```python
from build123d import *

# Parameters (mm, degrees)
CUT_EXTRUDE1_DEPTH  = 2
CUT_EXTRUDE1_DRAFT  = -12
SKETCH3_R           = 1.5
BOSS_EXTRUDE1_DEPTH = 36


with BuildPart() as part:
    # Sketch1 → Revolve2 (revolve)
    with BuildSketch(Plane(origin=(0, 0, 0), x_dir=(1, 0, 0), z_dir=(0, 1, 0))):
        with BuildLine():
            Line((0, 0), (0, 2))
            Line((0, 2), (1.798285661, 2))
            ThreePointArc((1.798285661, 2), (1.941964308, 1.978911731), (2.07352322, 1.917425786))
            ThreePointArc((2.07352322, 1.917425786), (2.674697589, 1.044998208), (2.5, 0))
            Line((2.5, 0), (0, 0))
        make_face()
    revolve(axis=Axis((0, 0, -0.65925001), (0, 0, -1)))


with BuildPart() as cut_extrude1_tool:
    # Sketch2 → Cut-Extrude1 (with draft: the straight prism first)
    with BuildSketch(Plane(origin=(0, 0, -2), x_dir=(-1, 0, 0), z_dir=(0, 0, -1))):
        Polygon((0.5, -0.5), (2, -0.5), (2, 0.5), (0.5, 0.5), (0.5, 2), (-0.5, 2), (-0.5, 0.5), (-2, 0.5), (-2, -0.5), (-0.5, -0.5), (-0.5, -2), (0.5, -2), align=None)
    extrude(amount=-CUT_EXTRUDE1_DEPTH)
    # Cut-Extrude1: the draft: its side faces are tilted about the plane it starts from
    cut_extrude1_sides = [cut_extrude1_tool.faces().sort_by_distance(p)[0] for p in [
        (-1.25, -0.5, -1),
        (-2, 0, -1),
        (-1.25, 0.5, -1),
        (-0.5, 1.25, -1),
        (0, 2, -1),
        (0.5, 1.25, -1),
        (1.25, 0.5, -1),
        (2, 0, -1),
        (1.25, -0.5, -1),
        (0.5, -1.25, -1),
        (0, -2, -1),
        (-0.5, -1.25, -1),
    ]]
    draft(cut_extrude1_sides, Plane(origin=(0, 0, -2), x_dir=(-1, 0, 0), z_dir=(0, 0, -1)), CUT_EXTRUDE1_DRAFT)


with BuildPart() as part_1:
    add(part.part)

    # Cut-Extrude1: cut by cut_extrude1_tool
    add(cut_extrude1_tool.part, mode=Mode.SUBTRACT)

    # Sketch3 → Boss-Extrude1 (add)
    with BuildSketch(Plane.XY):
        with Locations(Location((0.013589602, -0.013589602, 0), (0, 0, 182.342035556))):
            Circle(SKETCH3_R)
    extrude(amount=BOSS_EXTRUDE1_DEPTH)


solid = part_1.part
```
The model under review builds one solid part; all positions refer to its coordinate system, in mm. A direction names the side the tool comes from. Coordinates: 2 decimals unless noted, no trailing zeros. Write each loop counter-clockwise with the first axis right and the second up, starting at its lowest first coordinate (ties: lowest second). Pieces come first, ordered by that corner, then holes. Notation, with made-up numbers: (60, 64.25) - (69, 64.25) arc R34 ccw to (69, 94.25) - close; hole circle Ø2 at (-29.75, -37.75). An arc over 180 degrees is marked (long way). Answer in a Markdown table with one row per item. Add a question column.
Q1. Draft analysis for pull direction X (two halves, no side actions). For faces 1 (the face through (-1.4, -0.52, 17.75)), 2 (the face through (0.29, -1.02, -1.01)), 3 (the face through (1, 1, -2)), state which applies: +X half, -X half, draft (parallel to the pull), parting line (faces both ways), or undercut.
Q2. To check wall thickness, follow line 1 along Z through (x, y) = (1, -1.7); line 2 along Y through (x, z) = (-1, 15.5); line 3 along Y through (x, z) = (1.2, 0.5). State the ranges of each line that lie inside material, in increasing order. Write a range as from..to.
Q3. Clearance check with flat-ended pins moving along their axes: pin 1 (1 mm diameter, centred on x = -0.5, z = 20.5, fed in from +Y); pin 2 (2 mm diameter, centred on y = 1.5, z = 29, fed in from -X); pin 3 (1 mm diameter, centred on x = 2, y = -1.5, fed in from +Z). State where each tip first meets the part, or that it passes through.
Q4. For faces 4 (the face through (0, 0, 36)), 5 (the face through (2, 0, 0)), 6 (the face through (1.04, -0.29, -1.01)), list the 3-axis set-ups (+Z, -Z, +X, -X, +Y, -Y) from which the entire face can be reached by the end or side of a thin tool; tool diameter is ignored.
Q5. Consider section A-A on z = 2. Give the boundary of the cut face in (x, y).
Answers below:
| question | item | result |
|---|---|---|
| 1 | face 1 | parting line |
| 1 | face 2 | undercut |
| 1 | face 3 | draft |
| 2 | line 1 | -1.97..0 |
| 2 | line 2 | -1.12..1.09 |
| 2 | line 3 | -0.93..0.9 |
| 3 | pin 1 | y = 1.49 |
| 3 | pin 2 | x = -1.4 |
| 3 | pin 3 | z = 0 |
| 4 | face 4 | +Z, +X, -X, +Y, -Y |
| 4 | face 5 | +Z |
| 4 | face 6 | -Z |
| 5 | outline | circle Ø3 at (0.01, -0.01) |
